Input: part model. Units: mm. Frame: model coordinates. Face numbers are marked on the shaded views. A direction names the side the tool comes from. Give positions to 0.01 mm unless a question says otherwise; leave off trailing zeros. Loops run counter-clockwise (first coordinate to the right, second up) from the corner with the lowest first, then second, coordinate; pieces in that order, holes last. Notation, with made-up numbers: (-14.75, 82) - (10.25, 82) arc R24 ccw to (10.25, 104) - close; hole circle Ø1 at (-40, 34.5). An arc over 180 degrees is marked (long way). Answer as a JSON object with one key per item and string values. Group by question number.
(1) Mould query, pull axis Z, two halves, no side actions, for the marked faces 4, 5 and 6. Classes: +Z half, -Z half, draft (parallel to the pull), parting line (faces both ways), or undercut.
(2) Pin query (flat end, axial travel): P1, Ø10, axis at y = 1, z = -1.5, coming from the -X side; P2, Ø2, axis at x = 15.5, z = -0.5, coming from the +Y side; P3, Ø1.5, axis at y = -5, z = -3.5, coming from the +X side; P4, Ø1.5, axis at x = 5, z = -6.5, coming from the -Y side. Return the tip coordinate at first contact, or that it passes through.
(3) Material intervals for L1, parallel to Z at x = -1.2, y = 0; L2, parallel to X at y = -6.75, z = -1.75, sorted ascending.
(4) Section query C-C (x = 19.5). Return loops of the section in (y, z), plus the area to 3 significant figures.
(5) Section query D-D (z = 4.75). Count the separate pieces of the cut face and the enclosed holes in it, plus the area to 3 significant figures.
(6) Access query for the marked faces 1, 2 and 3. Directions: +Z, -Z, +X, -X, +Y, -Y. A direction counts if a zero-diameter tool reaches every point of the face in a straight line with its end or side. Return the directions, or none.
```python
from build123d import *

# Parameters (mm, degrees)
M2_CLEARANCE_HOLE2_D = 2.4
CHAMFER2_SIZE        = 0.25
CUT_EXTRUDE1_START   = 2
CUT_EXTRUDE1_DEPTH   = 26.002314716
FILLET1_R            = 0.25


with BuildPart() as part:
    # Sketch1 → Revolve1 (revolve)
    with BuildSketch(Plane.XY):
        with BuildLine():
            Line((0, 0), (0, 8))
            ThreePointArc((0, 8), (-0.125, 8.216506351), (-0.375, 8.216506351))
            Line((-0.375, 8.216506351), (-0.75, 8))
            Line((-0.75, 8), (-2.5, 8))
            Line((-2.5, 8), (-2.5, 8.75))
            Line((-2.5, 8.75), (3, 8.75))
            Line((3, 8.75), (3, 4))
            Line((3, 4), (14, 4))
            Line((14, 4), (14, 3))
            Line((14, 3), (24, 3))
            Line((24, 3), (24, 0))
            Line((24, 0), (0, 0))
        make_face()
    revolve(axis=Axis((24, 0, 0), (-1, 0, 0)))

    # M2 Clearance Hole2 (through all)
    with Locations(Plane(origin=(3, 0, 0), x_dir=(0, 0, -1), z_dir=(1, 0, 0))):
        with Locations((4.242640687, 4.242640687), (-4.242640687, 4.242640687), (4.242640687, -4.242640687), (-4.242640687, -4.242640687)):
            Hole(M2_CLEARANCE_HOLE2_D / 2)

    # Chamfer2
    chamfer2_edges = [part.edges().sort_by_distance(p)[0] for p in [
        (3, -8.75, 0),
        (14, -4, 0),
        (24, -3, 0),
    ]]
    chamfer(chamfer2_edges, length=CHAMFER2_SIZE)

    # Sketch5 → Cut-Extrude1 (cut, through all)
    with BuildSketch(Plane(origin=(0, 0, 0), x_dir=(1, 0, 0), z_dir=(0, 1, 0)).offset(CUT_EXTRUDE1_START)):
        with BuildLine():
            Line((13, 1), (18, 1))
            ThreePointArc((18, 1), (19, 0), (18, -1))
            Line((18, -1), (13, -1))
            ThreePointArc((13, -1), (12, 0), (13, 1))
        make_face()
    extrude(amount=CUT_EXTRUDE1_DEPTH, mode=Mode.SUBTRACT)

    # Fillet1
    fillet1_edges = [part.edges().sort_by_distance(p)[0] for p in [
        (3, -4, 0),
    ]]
    fillet(fillet1_edges, radius=FILLET1_R)


solid = part.part
```
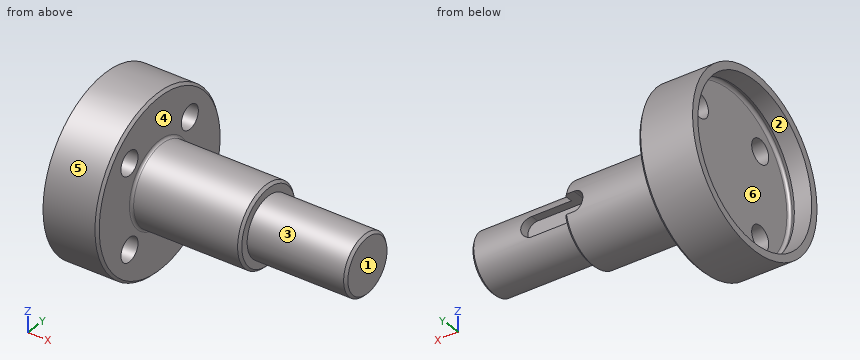
Recorded:
{
 "1": {"face 4": "draft", "face 5": "parting line", "face 6": "undercut"},
 "2": {"P1": "stops at x = 0", "P2": "stops at y = 2.83", "P3": "stops at x = 3", "P4": "passes through"},
 "3": {"L1": "z = -8.75 to -8, 8 to 8.75", "L2": "x = 0 to 3"},
 "4": {"outline": "circle Ø6 at (0, 0)", "area": "28.3 mm^2"},
 "5": {"separate pieces": "3", "enclosed holes": "0", "area": "35.2 mm^2"},
 "6": {"face 1": "+Z, -Z, +X, +Y, -Y", "face 2": "-X", "face 3": "+X"}
}
